Geometry: see drawing. Coordinates: mm, zero at the bounding-box minimum. Give positions to 0.01 mm unless a question says otherwise; leave off trailing zeros. Write each loop counter-clockwise with the first axis right and the second up, starting at its lowest first coordinate (ties: lowest second). Pieces come first, ordered by that corner, then holes. Notation, with made-up numbers: M 70.25,83.5 L 91.25,83.5 A30 cw 91.25,122.5 Z; hole C -10.75,-6 d5. An arc over 180 degrees is marked long. Use a Markdown table: item, result. Add a question column.
1) Section B-B on y = 10.5. State how many separate pieces and enclosed holes the cut face has, then the cut area to 3 significant figures.
2) Line query: line 1 (X direction, y = 7.75, z = 50.8); line 2 (X direction, y = 4.75, z = 51.5); line 3 (Z direction, x = 89.5, y = 11) (1 decimal). Output: solid intervals per line, ascending.
3) Section A-A on z = 50.8. Return the cut outline in (x, y).
4) Section D-D on z = 12.5. Return the cut outline in (x, y), then the cut area to 3 significant figures.
5) Draft query along X for the marked faces 1, 2 and 3. Return one class per face: +X half, -X half, draft (parallel to the pull), parting line (faces both ways), or undercut.
6) Section C-C on x = 88.9. Return the cut outline in (y, z), then the cut area to 3 significant figures.
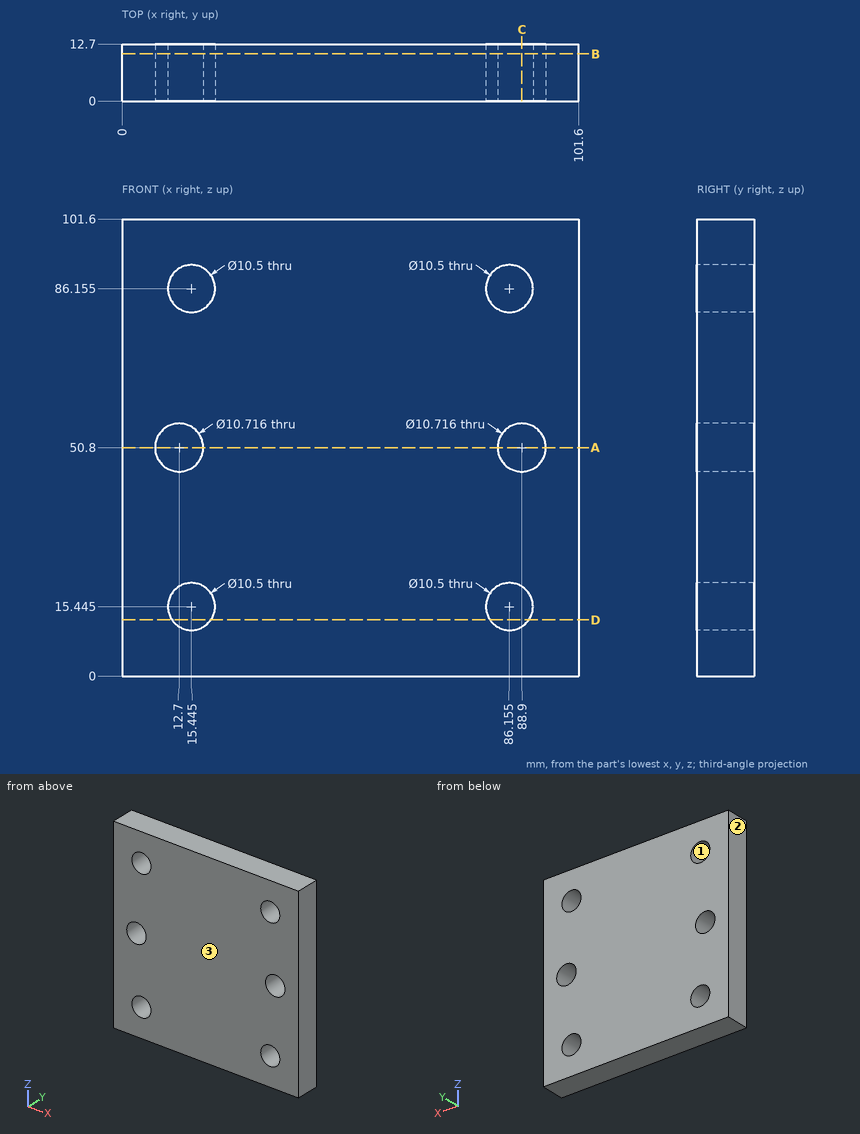
Found:
| question | item | result |
|---|---|---|
| 1 | separate pieces | 1 |
| 1 | enclosed holes | 6 |
| 1 | area | 9,800 mm² |
| 2 | line 1 | 0 to 7.34, 18.06 to 83.54, 94.26 to 101.6 |
| 2 | line 2 | 0 to 7.39, 18.01 to 83.59, 94.21 to 101.6 |
| 2 | line 3 | 0 to 11.4, 19.5 to 45.5, 56.1 to 82.1, 90.2 to 101.6 |
| 3 | outline | M 0,0 L 7.34,0 L 7.34,12.7 L 0,12.7 Z; M 18.06,0 L 83.54,0 L 83.54,12.7 L 18.06,12.7 Z; M 94.26,0 L 101.6,0 L 101.6,12.7 L 94.26,12.7 Z |
| 4 | outline | M 0,0 L 11.1,0 L 11.1,12.7 L 0,12.7 Z; M 19.79,0 L 81.81,0 L 81.81,12.7 L 19.79,12.7 Z; M 90.5,0 L 101.6,0 L 101.6,12.7 L 90.5,12.7 Z |
| 4 | area | 1,070 mm² |
| 5 | face 1 | undercut |
| 5 | face 2 | -X half |
| 5 | face 3 | draft |
| 6 | outline | M 0,0 L 12.7,0 L 12.7,10.97 L 0,10.97 Z; M 0,19.92 L 12.7,19.92 L 12.7,45.44 L 0,45.44 Z; M 0,56.16 L 12.7,56.16 L 12.7,81.68 L 0,81.68 Z; M 0,90.63 L 12.7,90.63 L 12.7,101.6 L 0,101.6 Z |
| 6 | area | 927 mm² |
